Work out the finished part from the listing and answer in its coordinate system (mm). A direction names the side the tool comes from. Coordinates: 2 decimals unless noted, no trailing zeros. Use a Markdown table: item, result.
from build123d import *

# Parameters (mm, degrees)
BOSS_EXTRUDE1_DEPTH      = 10
BOSS_EXTRUDE1_DEPTH_BACK = 10
SKETCH2_R                = 3
BOSS_EXTRUDE2_DEPTH      = 1.5
BOSS_EXTRUDE2_DEPTH_BACK = 2.5
SKETCH3_R                = 15.7
BOSS_EXTRUDE4_START      = 10
SKETCH4_R                = 15.7
SKETCH4_R_2              = 12.7
BOSS_EXTRUDE4_DEPTH      = 10
FILLET6_R                = 0.5
CHAMFER1_SIZE            = 0.5
SKETCH5_R                = 19.89902312
SKETCH5_R_2              = 15.7
SKETCH5_R_3              = 14.7
CUT_EXTRUDE2_DEPTH       = 135.083701085
FILLET7_R                = 0.2
CHAMFER3_SIZE            = 1


with BuildPart() as part:
    # Sketch2 → Boss-Extrude1 (new, two sides: drawn at the far end of the back side and taken through both)
    with BuildSketch(Plane.XY.offset(-BOSS_EXTRUDE1_DEPTH_BACK)):
        with BuildLine():
            Line((94.051269644, 47.422261979), (89.989154813, 58.054980417))
            Line((89.989154813, 58.054980417), (104.935548085, 63.765087962))
            Line((104.935548085, 63.765087962), (108.997662915, 53.132369524))
            ThreePointArc((108.997662915, 53.132369524), (104.379520052, 42.804119115), (94.051269644, 47.422261979))
        make_face()
        with Locations((101.52446628, 50.277315751)):
            Circle(SKETCH2_R, mode=Mode.SUBTRACT)
    extrude(amount=BOSS_EXTRUDE1_DEPTH + BOSS_EXTRUDE1_DEPTH_BACK)

    # Sketch3 → Boss-Extrude2 (add, two sides: drawn at the far end of the back side and taken through both)
    with BuildSketch(Plane(origin=(-7.892992814, 20.660166865, 0), x_dir=(0.9341495794706384, 0.3568817215476715, 0), z_dir=(-0.3568817215476715, 0.9341495794706384, 0)).offset(-BOSS_EXTRUDE2_DEPTH_BACK)):
        with Locations(Location((112.782092481, 0, 0), (0, 0, 180))):
            Circle(SKETCH3_R)
    extrude(amount=BOSS_EXTRUDE2_DEPTH + BOSS_EXTRUDE2_DEPTH_BACK)

    # Sketch4 → Boss-Extrude4 (add)
    with BuildSketch(Plane(origin=(-8.428315397, 22.061391234, 0), x_dir=(0.9341495794706381, 0.3568817215476716, 0), z_dir=(-0.3568817215476716, 0.9341495794706383, 0)).offset(BOSS_EXTRUDE4_START)):
        with Locations(Location((112.782092481, 0, 0), (0, 0, 180))):
            Circle(SKETCH4_R)
        with Locations(Location((112.782092481, 0, 0), (0, 0, 180))):
            Circle(SKETCH4_R_2, mode=Mode.SUBTRACT)
    extrude(amount=-BOSS_EXTRUDE4_DEPTH)

    # Fillet6
    fillet6_edges = [part.edges().sort_by_distance(p)[0] for p in [
        (104.379520052, 42.804119115, 10),
        (107.412707652, 57.281041768, 10),
        (92.46631438, 51.570934224, 10),
        (92.46631438, 51.570934224, -10),
        (104.379520052, 42.804119115, -10),
        (107.412707652, 57.281041768, -10),
    ]]
    fillet(fillet6_edges, radius=FILLET6_R)

    # Chamfer1
    chamfer1_edges = [part.edges().sort_by_distance(p)[0] for p in [
        (98.52446628, 50.277315751, -10),
        (98.52446628, 50.277315751, 10),
    ]]
    chamfer(chamfer1_edges, length=CHAMFER1_SIZE)

    # Sketch5 → Cut-Extrude2 (cut, through all)
    # profile 1 of 2: a face of its own
    with BuildSketch(Plane(origin=(-11.997132612, 31.402887029, 0), x_dir=(0.9341495794706383, 0.35688172154767156, 0), z_dir=(-0.35688172154767156, 0.9341495794706383, 0))):
        with Locations((112.782092481, 0)):
            Circle(SKETCH5_R)
        with Locations((112.782092481, 0)):
            Circle(SKETCH5_R_2, mode=Mode.SUBTRACT)
    # profile 2 of 2: a face of its own
    with BuildSketch(Plane(origin=(-11.997132612, 31.402887029, 0), x_dir=(0.9341495794706383, 0.35688172154767156, 0), z_dir=(-0.35688172154767156, 0.9341495794706383, 0))):
        with Locations((112.782092481, 0)):
            Circle(SKETCH5_R_2)
        with Locations(Location((112.782092481, 0, 0), (0, 0, 180))):
            Circle(SKETCH5_R_3, mode=Mode.SUBTRACT)
    extrude(amount=-CUT_EXTRUDE2_DEPTH, mode=Mode.SUBTRACT)

    # Fillet7
    fillet7_edges = [part.edges().sort_by_distance(p)[0] for p in [
        (105.22191131, 76.185152217, 0),
        (107.090210469, 76.89891566, 0),
    ]]
    fillet(fillet7_edges, radius=FILLET7_R)

    # Chamfer3
    chamfer3_edges = [part.edges().sort_by_distance(p)[0] for p in [
        (105.827752388, 61.429714013, 0),
        (98.354555753, 58.574660241, -10),
        (90.881359117, 55.719606469, 0),
        (98.354555753, 58.574660241, 10),
        (105.69094935, 61.377449895, -9.853553391),
        (91.018162155, 55.771870587, -9.853553391),
        (105.69094935, 61.377449895, 9.853553391),
        (91.018162155, 55.771870587, 9.853553391),
        (112.086554571, 63.820821548, 0),
    ]]
    chamfer(chamfer3_edges, length=CHAMFER3_SIZE)


solid = part.part
(1) Given P1, Ø1.5, axis at x = 88, z = -2, coming from the -Y side; P2, Ø2, axis at y = 51, z = 1, coming from the -X side; P3, Ø5.5, axis at x = 101.52, y = 50.28, coming from the +Z side; P4, Ø5, axis at x = 98.5, y = 49, coming from the -Z side, each flat-ended and moving along its own axis, determine where each tip first touches the part or whether it passes through.
Conclusion:
| item | result |
|---|---|
| P1 | y = 54.33 |
| P2 | x = 92.3 |
| P3 | through |
| P4 | z = -10 |
(2) Straight lines are drawn through the part: L1, parallel to Z at x = 98, y = 54.5; L2, parallel to Z at x = 96, y = 63.5; L3, parallel to Y at x = 100.5, z = 2.25. For each, find the intervals that lie inside material, in ascending order.
Conclusion:
| item | result |
|---|---|
| L1 | -10 to 10 |
| L2 | -14.69 to -12.69, 12.69 to 14.69 |
| L3 | 42.34 to 47.46, 53.1 to 63.68 |
(3) Which of the six approach directions +Z, -Z, +X, -X, +Y, -Y give full straight-line access (tool end or side, diameter ignored) to faces 5 (the flat face through (99, 54, -10)), 6 (the flat face through (97.093, 62.375, 0.178)), 7 (the cylindrical face through (107.47, 56.71, 9.86)), 8 (the flat face through (107.57, 56.87, -0.13))?
Conclusion:
| item | result |
|---|---|
| face 5 | -Z, +X, -Y |
| face 6 | none |
| face 7 | +Z, +X |
| face 8 | +Z, -Z, +X |
(4) Determine the mould class of faces 1 (the flat face through (90.6, 55.07, 0.13)), 2 (the cylindrical face through (99.31, 52.3, -0.13)), 3 (the cylindrical face through (92.77, 51.21, 9.86)), 4 (the flat face through (98.44, 58.06, -10.49)) for opening direction X: pulls with the +X half, pulls with the -X half, needs draft (parallel to the pull), parting line crosses it, or undercut.
Conclusion:
| item | result |
|---|---|
| face 1 | undercut |
| face 2 | undercut |
| face 3 | pulls with the -X half |
| face 4 | pulls with the +X half |
